Geometry: see drawing. Coordinates: mm, zero at the bounding-box minimum. Give positions to 0.01 mm unless a question says otherwise; leave off trailing zeros. Write each loop counter-clockwise with the first axis right and the second up, starting at its lowest first coordinate (ties: lowest second). Pieces come first, ordered by that corner, then holes. Notation, with made-up numbers: (31.25, 75.25) -> (65.25, 75.25) arc R15 cw to (65.25, 86.25) -> close; hole circle Ø5 at (89, 28). An arc over 180 degrees is marked (long way). Write item = value, one per line.
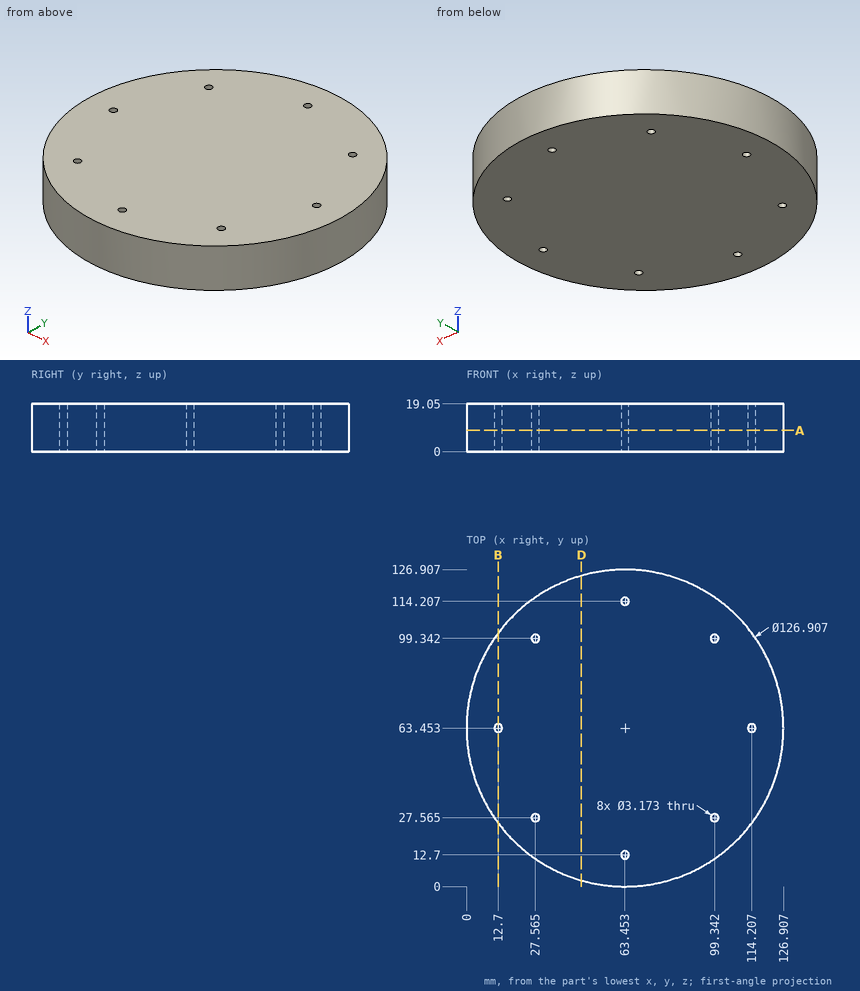
(1) Section query A-A (z = 8.5). Give the number of separate pieces and of enclosed holes in the cut face, plus the area to 3 significant figures.
Values follow:
separate_pieces = 1
enclosed_holes = 8
area = 12,600 mm2
(2) Section query D-D (x = 46). Return loops of the section in (y, z), plus the area to 3 significant figures.
Values follow:
outline = (2.45, 0) -> (124.46, 0) -> (124.46, 19.05) -> (2.45, 19.05) -> close
area = 2,320 mm2
(3) Section query B-B (x = 12.7). Return loops of the section in (y, z).
Values follow:
outline = (25.37, 0) -> (61.87, 0) -> (61.87, 19.05) -> (25.37, 19.05) -> close; (65.04, 0) -> (101.54, 0) -> (101.54, 19.05) -> (65.04, 19.05) -> close
(4) Material intervals for line 1 (X direction, y = 62, z = 9) (1 decimal); line 2 (Y direction, x = 99, z = 2) (1 decimal), sorted ascending.
Values follow:
line_1 = 0 to 12.1, 13.3 to 113.6, 114.8 to 126.9
line_2 = 10.9 to 26, 29.1 to 97.8, 100.9 to 116
(5) First-contact query: pin 1 (3 mm diameter, centred on x = 63.45, y = 12.7, fed in from -Z); pin 2 (6 mm diameter, centred on x = 50, z = 3.5, fed in from -Y); pin 3 (1 mm diameter, centred on y = 65, z = 7, fed in from -X); pin 4 (2 mm diameter, centred on x = 56.5, z = 12, fed in from +Y). Flat tips, straight axial feed; report the tip coordinate or a pass-through.
Values follow:
pin_1 = through
pin_2 = 0.87
pin_3 = 0.01
pin_4 = 126.63
